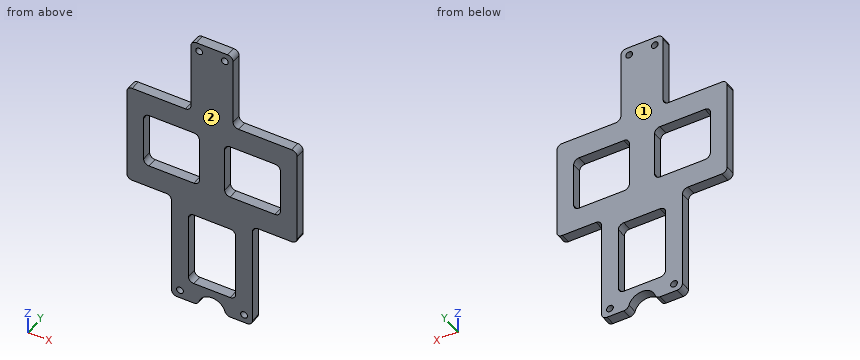
```python
from build123d import *

# Parameters (mm, degrees)
SKETCH1_W                    = 79.6544
SKETCH1_H                    = 135.6868
BOSS_EXTRUDE1_DEPTH          = 4.6482
SKETCH2_W                    = 20.9042
SKETCH2_H                    = 51.435
SKETCH2_W_2                  = 22.098
SKETCH2_H_2                  = 35.56
SKETCH2_W_3                  = 26.0477
SKETCH2_H_3                  = 26.1112
SKETCH2_W_4                  = 29.9593
SKETCH2_H_4                  = 36.4998
CUT_EXTRUDE1_DEPTH           = 79.806970165
F_1_8_0_125_DIAMETER_HOLE1_D = 3.175
FILLET1_R                    = 2.54


with BuildPart() as part:
    # Sketch1 → Boss-Extrude1 (new body)
    with BuildSketch(Plane(origin=(0, 0, 0), x_dir=(1, 0, 0), z_dir=(0, 1, 0))):
        Rectangle(SKETCH1_W, SKETCH1_H)
    extrude(amount=BOSS_EXTRUDE1_DEPTH)

    # Sketch2 → Cut-Extrude1 (cut, through all)
    with BuildSketch(Plane(origin=(0, 4.6482, 0), x_dir=(1, 0, 0), z_dir=(0, 1, 0))):
        with Locations((29.3751, 42.1259)):
            Rectangle(SKETCH2_W, SKETCH2_H)
        with Locations((0, 39.9034)):
            Rectangle(SKETCH2_W_2, SKETCH2_H_2)
        with Locations((18.92935, -7.493)):
            Rectangle(SKETCH2_W_3, SKETCH2_H_3)
        with Locations((-18.92935, -7.493)):
            Rectangle(SKETCH2_W_3, SKETCH2_H_3)
        with Locations((-24.84755, -49.5935)):
            Rectangle(SKETCH2_W_4, SKETCH2_H_4)
        with Locations((24.84755, -49.5935)):
            Rectangle(SKETCH2_W_4, SKETCH2_H_4)
        with BuildLine():
            Line((6.35, 67.8434), (-6.35, 67.8434))
            ThreePointArc((-6.35, 67.8434), (0, 61.4934), (6.35, 67.8434))
        make_face()
        with BuildLine():
            ThreePointArc((6.35, 67.8434), (0, 74.1934), (-6.35, 67.8434))
            Line((-6.35, 67.8434), (6.35, 67.8434))
        make_face()
        with Locations((-29.3751, 42.1259)):
            Rectangle(SKETCH2_W, SKETCH2_H)
    extrude(amount=-CUT_EXTRUDE1_DEPTH, mode=Mode.SUBTRACT)

    # 1/8 (0.125) Diameter Hole1 (through all)
    with Locations(Plane(origin=(-14.9733, 4.6482, -63.9445), x_dir=(0, 0, 1), z_dir=(0, 1, 0))):
        with Locations((0, 0), (0, 29.9466), (127.889, 20.96135), (127.889, 8.98525)):
            Hole(F_1_8_0_125_DIAMETER_HOLE1_D / 2)

    # Fillet1
    fillet1_edges = [part.edges().sort_by_distance(p)[0] for p in [
        (-9.8679, 2.3241, 67.8434),
        (-39.8272, 2.3241, 31.3436),
        (-9.8679, 2.3241, 31.3436),
        (-5.9055, 2.3241, -5.5626),
        (-5.9055, 2.3241, 20.5486),
        (-31.9532, 2.3241, 20.5486),
        (-31.9532, 2.3241, -5.5626),
        (31.9532, 2.3241, -5.5626),
        (31.9532, 2.3241, 20.5486),
        (5.9055, 2.3241, 20.5486),
        (5.9055, 2.3241, -5.5626),
        (11.049, 2.3241, -22.1234),
        (-11.049, 2.3241, -22.1234),
        (-11.049, 2.3241, -57.6834),
        (11.049, 2.3241, -57.6834),
        (9.8679, 2.3241, 67.8434),
        (9.8679, 2.3241, 31.3436),
        (39.8272, 2.3241, 31.3436),
        (-6.35, 2.3241, -67.8434),
        (6.35, 2.3241, -67.8434),
        (-18.923, 2.3241, -67.8434),
        (-18.923, 2.3241, -16.4084),
        (-39.8272, 2.3241, -16.4084),
        (18.923, 2.3241, -67.8434),
        (39.8272, 2.3241, -16.4084),
        (18.923, 2.3241, -16.4084),
    ]]
    fillet(fillet1_edges, radius=FILLET1_R)


solid = part.part
```
Part model, mm, in its own coordinate system. Face numbers are marked on the shaded views. Give positions to 0.01 mm unless a question says otherwise; leave off trailing zeros. Write each loop counter-clockwise with the first axis right and the second up, starting at its lowest first coordinate (ties: lowest second). Pieces come first, ordered by that corner, then holes. Notation, with made-up numbers: (89.5, -24) -> (130.5, -24) arc R20 ccw to (130.5, 4) -> close; hole circle Ø5 at (42, 45). An arc over 180 degrees is marked (long way). Put each result on its own line as item: value. Start each with the question number.
Item 1: Cut at B-B (z = 13). List the corners of the cut face in (x, y), then the cut area to 3 significant figures.
Item 2: Cut at A-A (z = -45). List the corners of the cut face in (x, y), then the cut area to 3 significant figures.
Item 3: Cut at D-D (x = -34). List the corners of the cut face in (y, z), then the cut area to 3 significant figures.
Item 4: Wall check: L1, parallel to X at y = 0.25, z = -55.5; L2, parallel to Z at x = -0.5, y = 4.4; L3, parallel to X at y = 1.9, z = 8.5. Give the ranges that are in metal, low to high. Write a range as [from, to].
Item 5: Pin check, flat tips, straight feed: pin 1 Ø2.5 at (x, y) = (-21, 3.5) entering from -Z; pin 2 Ø1.4 at (y, z) = (3, 45.5) entering from -X; pin 3 Ø4 at (x, z) = (14.97, -63.94) entering from -Y; pin 4 Ø2.5 at (x, y) = (-22, 3) entering from +Z. Stop position of each tip, or through.
Item 6: Cut at C-C (x = -23). List the corners of the cut face in (y, z), then the cut area to 3 significant figures.
Item 7: Pull direction Y, two halves, no side cores. Call the marked faces 1 and 2: pulls with the +Y half, pulls with the -Y half, needs draft (parallel to the pull), parting line crosses it, or undercut.
Answer list:
1. outline: (-39.83, 0) -> (-31.95, 0) -> (-31.95, 4.65) -> (-39.83, 4.65) -> close; (-5.91, 0) -> (5.91, 0) -> (5.91, 4.65) -> (-5.91, 4.65) -> close; (31.95, 0) -> (39.83, 0) -> (39.83, 4.65) -> (31.95, 4.65) -> close
1. area: 128 mm2
2. outline: (-18.92, 0) -> (-11.05, 0) -> (-11.05, 4.65) -> (-18.92, 4.65) -> close; (11.05, 0) -> (18.92, 0) -> (18.92, 4.65) -> (11.05, 4.65) -> close
2. area: 73.2 mm2
3. outline: (0, -16.41) -> (4.65, -16.41) -> (4.65, 31.34) -> (0, 31.34) -> close
3. area: 222 mm2
4. L1: x = [-18.92, -11.02], [11.02, 18.92]
4. L2: z = [-61.51, -57.68], [-22.12, 67.84]
4. L3: x = [-39.83, -31.95], [-5.91, 5.91], [31.95, 39.83]
5. pin 1: stops at z = -17.07
5. pin 2: stops at x = -9.87
5. pin 3: stops at y = 0
5. pin 4: stops at z = 31.34
6. outline: (0, -16.41) -> (4.65, -16.41) -> (4.65, -5.56) -> (0, -5.56) -> close; (0, 20.55) -> (4.65, 20.55) -> (4.65, 31.34) -> (0, 31.34) -> close
6. area: 101 mm2
7. face 1: pulls with the +Y half
7. face 2: pulls with the -Y half
